Geometry: final body of the model. Coordinates: model frame, mm. A direction names the side the tool comes from. Coordinates: 2 decimals unless noted, no trailing zeros. Write each loop counter-clockwise with the first axis right and the second up, starting at its lowest first coordinate (ties: lowest second). Pieces come first, ordered by that corner, then holes. Notation, with made-up numbers: (11.5, 10) - (29.5, 10) arc R20 ccw to (29.5, 15) - close; hole circle Ø7 at (4.5, -34.5). An arc over 180 degrees is marked (long way). Put each result on its own line as item: value.
```python
from build123d import *

# Parameters (mm, degrees)
BOSS_EXTRUDE1_DEPTH = 8
CHAMFER5_SIZE       = 5
FILLET1_R           = 2.5
SKETCH2_R           = 1.5
CUT_EXTRUDE1_DEPTH  = 47.658332589
SKETCH3_R           = 2
CUT_EXTRUDE2_DEPTH  = 44.200115741


with BuildPart() as part:
    # Sketch1 → Boss-Extrude1 (new, symmetric)
    with BuildSketch(Plane.XY):
        Polygon((-36, 0), (-21, 0), (-21, 20.5), (21, 20.5), (21, 0), (36, 0), (36, 2.5), (28, 2.5), (28, 25), (-28, 25), (-28, 2.5), (-36, 2.5), align=None)
    extrude(amount=BOSS_EXTRUDE1_DEPTH, both=True)

    # Chamfer5
    chamfer5_edges = [part.edges().sort_by_distance(p)[0] for p in [
        (-28, 25, 0),
        (28, 25, 0),
        (21, 0, 0),
        (-21, 0, 0),
    ]]
    chamfer(chamfer5_edges, length=CHAMFER5_SIZE)

    # Fillet1
    fillet1_edges = [part.edges().sort_by_distance(p)[0] for p in [
        (-28, 2.5, 0),
        (28, 2.5, 0),
    ]]
    fillet(fillet1_edges, radius=FILLET1_R)

    # Sketch2 → Cut-Extrude1 (cut, through all)
    with BuildSketch(Plane.XY.offset(8)):
        with Locations((-24.75, 14.475)):
            Circle(SKETCH2_R)
        with Locations((-24.75, 5.725)):
            Circle(SKETCH2_R)
        with Locations((24.75, 14.475)):
            Circle(SKETCH2_R)
        with Locations((24.75, 5.725)):
            Circle(SKETCH2_R)
    extrude(amount=-CUT_EXTRUDE1_DEPTH, mode=Mode.SUBTRACT)

    # Sketch3 → Cut-Extrude2 (cut, through all)
    with BuildSketch(Plane(origin=(0, 2.5, 0), x_dir=(1, 0, 0), z_dir=(0, 1, 0))):
        with Locations(Location((32.5, 4, 0), (0, 0, 270))):
            Circle(SKETCH3_R)
        with Locations(Location((32.5, -4, 0), (0, 0, 270))):
            Circle(SKETCH3_R)
        with Locations(Location((-32.5, 4, 0), (0, 0, 270))):
            Circle(SKETCH3_R)
        with Locations(Location((-32.5, -4, 0), (0, 0, 270))):
            Circle(SKETCH3_R)
    extrude(amount=-CUT_EXTRUDE2_DEPTH, mode=Mode.SUBTRACT)


solid = part.part
```
1. Section query D-D (z = 7). Return loops of the section in (x, y) (3 decimals), then the cut area to 3 significant figures.
Answer below:
outline: (-36, 0) - (-26, 0) - (-21, 5) - (-21, 20.5) - (21, 20.5) - (21, 5) - (26, 0) - (36, 0) - (36, 2.5) - (30.5, 2.5) arc R2.5 cw to (28, 5) - (28, 20) - (23, 25) - (-23, 25) - (-28, 20) - (-28, 5) arc R2.5 cw to (-30.5, 2.5) - (-36, 2.5) - close; hole circle Ø3 at (-24.75, 5.725); hole circle Ø3 at (-24.75, 14.475); hole circle Ø3 at (24.75, 5.725); hole circle Ø3 at (24.75, 14.475)
area: 503 mm²
2. Section query A-A (x = 32.5). Return loops of the section in (y, z), then the cut area to 3 significant figures.
Answer below:
outline: (0, -8) - (2.5, -8) - (2.5, -6) - (0, -6) - close; (0, -2) - (2.5, -2) - (2.5, 2) - (0, 2) - close; (0, 6) - (2.5, 6) - (2.5, 8) - (0, 8) - close
area: 20.0 mm²
3. Section query B-B (y = 10). Return loops of the section in (x, z).
Answer below:
outline: (-28, -8) - (-21, -8) - (-21, 8) - (-28, 8) - close; (21, -8) - (28, -8) - (28, 8) - (21, 8) - close
4. Mould query, pull axis Z, two halves, no side actions, for faces 1 (the flat face through (0, 22, -8)), 2 (the cylindrical face through (30.548, 1.268, 3.566)), 3 (the flat face through (-33, 2.5, 0)). Classes: +Z half, -Z half, draft (parallel to the pull), parting line (faces both ways), or undercut.
Answer below:
face 1: -Z half
face 2: undercut
face 3: draft
5. Pin query (flat end, axial travel): pin 1 Ø1.8 at (x, y) = (-24.75, 5.725) entering from -Z; pin 2 Ø6 at (x, z) = (34.5, 2) entering from +Y; pin 3 Ø4 at (y, z) = (17.5, 0) entering from +X; pin 4 Ø1 at (y, z) = (5, -0.5) entering from -X. Return the tip coordinate at first contact, or that it passes through.
Answer below:
pin 1: passes through
pin 2: stops at y = 2.5
pin 3: stops at x = 28
pin 4: stops at x = -28.05
6. Ray query, probe 1 along Z at (x, y) = (-32.5, 1.9); probe 2 along X at (y, z) = (10, -1); probe 3 along X at (y, z) = (1.25, 4). Return the intervals inside material, ascending. Write a range as from..to.
Answer below:
probe 1: z = -8..-6, -2..2, 6..8
probe 2: x = -28..-21, 21..28
probe 3: x = -36..-34.5, -30.5..-24.75, 24.75..30.5, 34.5..36
7. Section query C-C (x = 24.75). Return loops of the section in (y, z) (3 decimals).
Answer below:
outline: (1.25, -8) - (4.225, -8) - (4.225, 8) - (1.25, 8) - close; (7.225, -8) - (12.975, -8) - (12.975, 8) - (7.225, 8) - close; (15.975, -8) - (23.25, -8) - (23.25, 8) - (15.975, 8) - close
8. Set-up query: faces 4 (the cylindrical face through (-29, 3, 0)), 5 (the flat face through (-23, 3, 0)), 6 (the flat face through (28, 12, 0)). Return all of +Z, -Z, +X, -X, +Y, -Y with unobstructed straight access to the full face (end or side cutting, diameter ignored); none if empty.
Answer below:
face 4: +Z, -Z, -X, +Y
face 5: +Z, -Z, -Y
face 6: +Z, -Z, +X, +Y
